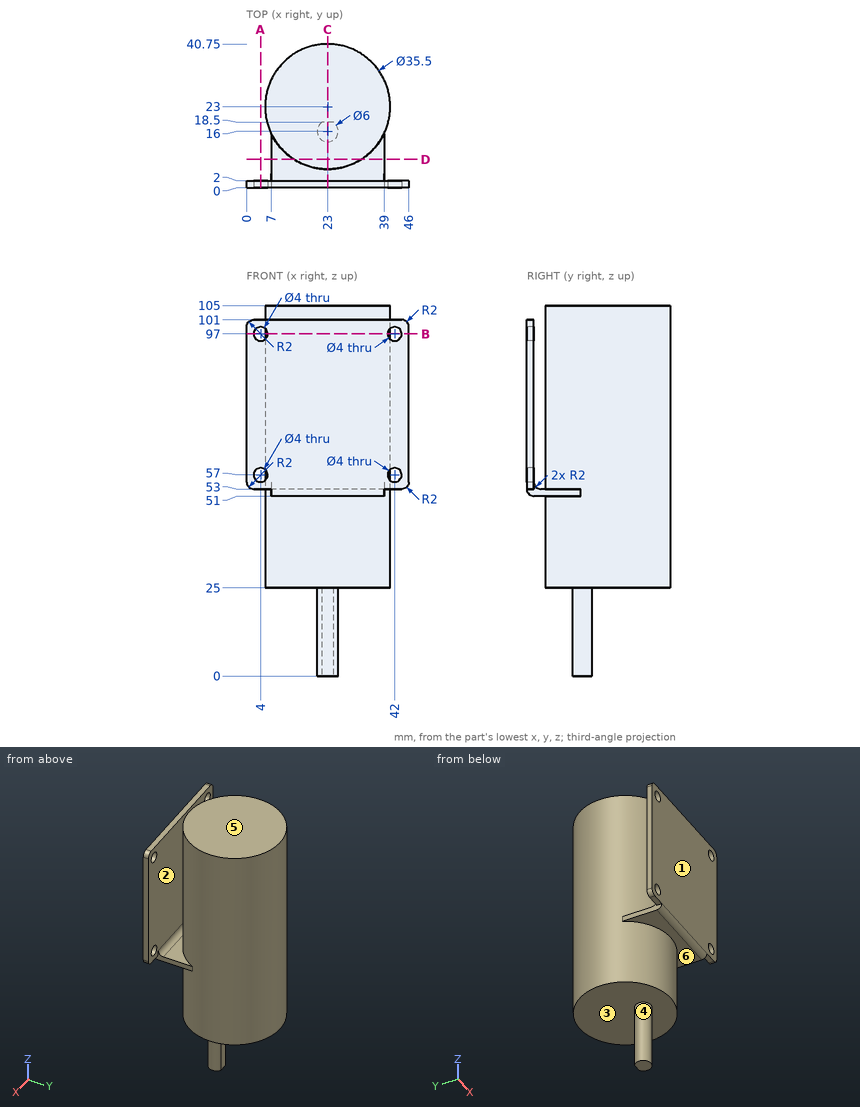
The figure shows three views and two pictorial views of one solid part (mm, origin at its lowest corner). Answer the questions. A direction names the side the tool comes from. Give positions to 0.01 mm unless a question says otherwise; leave off trailing zeros. Write each loop counter-clockwise with the first axis right and the second up, starting at its lowest first coordinate (ties: lowest second). Pieces come first, ordered by that corner, then holes. Notation, with made-up numbers: (-25, 1) - (-7, 1) arc R22 cw to (-7, 18) - close; hole circle Ø9 at (83, 32). An arc over 180 degrees is marked (long way). Use CSV: the item, a comma, the result in double quotes. Start each with the question number.
Item 1: The part is cut by section B-B, the plane z = 97. Give the vertices of the cut face in (x, y), and give its area (3 significant figures).
Item 2: Flat-ended cylindrical pins translate along their axes: P1, Ø1.5, axis at y = 9.5, z = 85.5, coming from the +X side; P2, Ø0.6, axis at x = 30, y = 1, coming from the +Z side; P3, Ø18, axis at x = 19.5, y = 32, coming from the -Z side. Find the tip coordinate at first contact, or state that the pin passes through.
Item 3: The mould has two halves that part along Y. Classify the marked faces 1, 2 and 3: pulls with the +Y half, pulls with the -Y half, needs draft (parallel to the pull), parting line crosses it, or undercut.
Item 4: The part is cut by section D-D, the plane y = 8. Give the vertices of the cut face in (x, z).
Item 5: The part is cut by section C-C, the plane x = 23. Give the vertices of the cut face in (y, z).
Item 6: The part is cut by section A-A, the plane x = 4. Give the vertices of the cut face in (y, z).
Item 7: For the marked faces 4, 5 and 6, determine the directions among +Z, -Z, +X, -X, +Y, -Y from which every point of the face is accessible in a straight line to the end or side of a thin tool.
Item 8: Consider line 1 (Z direction, x = 4, y = 1.45); line 2 (X direction, y = 0.7, z = 57); line 3 (Z direction, x = 29, y = 31). Determine where each line is inside the solid, lowest interval first.
Taken from the geometry:
1,outline,"(0, 0) - (2, 0) - (2, 2) - (0, 2) - close; circle Ø35.5 at (23, 23); (6, 0) - (40, 0) - (40, 2) - (6, 2) - close; (44, 0) - (46, 0) - (46, 2) - (44, 2) - close"
1,area,"1,070 mm2"
2,P1,"x = 35.35"
2,P2,"z = 101"
2,P3,"z = 25"
3,face 1,"pulls with the -Y half"
3,face 2,"undercut"
3,face 3,"needs draft"
4,outline,"(7, 51) - (13.51, 51) - (13.51, 25) - (32.49, 25) - (32.49, 51) - (39, 51) - (39, 53) - (32.49, 53) - (32.49, 105) - (13.51, 105) - (13.51, 53) - (7, 53) - close"
5,outline,"(0, 53) arc R2 ccw to (2, 51) - (5.25, 51) - (5.25, 25) - (13, 25) - (13, 0) - (18.5, 0) - (18.5, 25) - (40.75, 25) - (40.75, 105) - (5.25, 105) - (5.25, 53) - (4, 53) arc R2 cw to (2, 55) - (2, 101) - (0, 101) - close"
6,outline,"(0, 53) - (2, 53) - (2, 55) - (0, 55) - close; (0, 59) - (2, 59) - (2, 95) - (0, 95) - close; (0, 99) - (2, 99) - (2, 101) - (0, 101) - close"
7,face 4,"-Z"
7,face 5,"+Z, +X, -X, +Y, -Y"
7,face 6,"-Z, -Y"
8,line 1,"53 to 55, 59 to 95, 99 to 101"
8,line 2,"0 to 2, 6 to 40, 44 to 46"
8,line 3,"25 to 105"
